Model file for the job. Use its own axes, mm. A direction names the side the tool comes from. Coordinates: 2 decimals unless noted, no trailing zeros. Order: outer loops, then holes, each group sorted by start corner. A loop starts at its lowest first (then second) coordinate and runs counter-clockwise, first axis right, second up.
from build123d import *

# Parameters (mm, degrees)
F0_W     = 101.6
F0_H     = 152.4
F1_DEPTH = 127
F4_W     = 101.6
F4_H     = 76.2
F5_DEPTH = 63.5
F6_D     = 25.4


with BuildPart() as f1:
    # F0 (on Top) → F1 (new body)
    with BuildSketch(Plane.XY):
        with Locations((-6.65934, 45.666524)):
            Rectangle(F0_W, F0_H)
    extrude(amount=F1_DEPTH)

    # F4 (on face) → F5 (join)
    with BuildSketch(Plane(origin=(0, 121.866524, 0), x_dir=(-1, 0, 0), z_dir=(0, 1, 0))):
        with Locations((6.65934, 38.1)):
            Rectangle(F4_W, F4_H)
    extrude(amount=F5_DEPTH)

    # F6 (through all)
    with Locations(Plane.XZ.offset(30.533476)):
        with Locations((-4.961859, 38.326953)):
            Hole(F6_D / 2)


solid = f1.part
Q1. Which spindle directions (+Z, -Z, +X, -X, +Y, -Y) get a long thin tool onto all of the face, cutting with end or side? Do faces 5 (the face through (-7, 47, 127)), 6 (the face through (-7, 121.867, 101)). Say none if no direction does.
Established:
face 5: +Z, +X, -X, +Y, -Y
face 6: +Z, +X, -X, +Y
Q2. Cut at D-D, the plane x = 36.5. List the corners of the cut face in (y, z).
Established:
outline: (-30.53, 0) - (185.37, 0) - (185.37, 76.2) - (121.87, 76.2) - (121.87, 127) - (-30.53, 127) - close
Q3. Cut at A-A, the plane z = 33. List the corners of the cut face in (x, y).
Established:
outline: (-57.46, -30.53) - (-16.49, -30.53) - (-16.49, 185.37) - (-57.46, 185.37) - close; (6.57, -30.53) - (44.14, -30.53) - (44.14, 185.37) - (6.57, 185.37) - close
Q4. Cut at B-B, the plane x = 4.5. List the corners of the cut face in (y, z), plus the area to 3 significant figures.
Established:
outline: (-30.53, 0) - (185.37, 0) - (185.37, 29.86) - (-30.53, 29.86) - close; (-30.53, 46.8) - (185.37, 46.8) - (185.37, 76.2) - (121.87, 76.2) - (121.87, 127) - (-30.53, 127) - close
area: 20,500 mm2
Q5. Drop flat-ended pins along their axis: P1, Ø15, axis at x = -24, z = 100, coming from the +Y side; P2, Ø19, axis at x = -27, y = 150.5, coming from the +Z side. Give the stop position or say it passes through.
Established:
P1: stops at y = 121.87
P2: stops at z = 76.2
Q6. Probe line 1 (Y direction, x = -19.5, z = 103); line 2 (Z direction, x = -6.5, y = 69.5); line 3 (Z direction, x = 1.5, y = 89). List the from-to ranges inside material, lowest first.
Established:
line 1: y = -30.53 to 121.87
line 2: z = 0 to 25.72, 50.93 to 127
line 3: z = 0 to 27.39, 49.26 to 127
Q7. Cut at C-C, the plane y = 79. List the corners of the cut face in (x, z), plus the area to 3 significant figures.
Established:
outline: (-57.46, 0) - (44.14, 0) - (44.14, 127) - (-57.46, 127) - close; hole circle Ø25.4 at (-4.96, 38.33)
area: 12,400 mm2
Q8. Mould opens along X. For faces 1 (the face through (-3.31, 78.93, 50.92)), 2 (the face through (44.141, 52, 63)), 3 (the face through (-57.459, 52, 63)), 4 (the face through (5, 185.367, 47)) say: pulls with the +X half, pulls with the -X half, needs draft (parallel to the pull), parting line crosses it, or undercut.
Established:
face 1: undercut
face 2: pulls with the +X half
face 3: pulls with the -X half
face 4: needs draft
